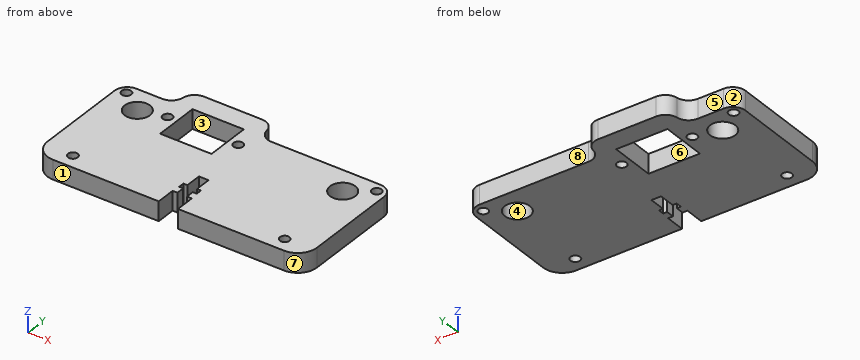
Autodesk Inventor part; units mm, degrees
ref_plane "YZ Plane" through (0, 0, 0) normal (1, 0, 0) x (0, 1, 0)
ref_plane "XZ Plane" through (0, 0, 0) normal (0, 1, 0) x (-1, 0, 0)
ref_plane "XY Plane" through (0, 0, 0) normal (0, 0, 1) x (1, 0, 0)
sketch "Sketch1" plane through (0, 0, 0) normal (0, 0, 1) x (1, 0, 0)
  arc A0 (-84, -33) -> (-78, -39) centre (-78, -33) ccw
  line L0 (-78, -39) -> (-45, -39)
  line L1 (-45, -39) -> (-45, -33)
  line L2 (-45, -33) -> (-43.5, -33)
  line L3 (-43.5, -33) -> (-43.5, -30.5)
  line L4 (-43.5, -30.5) -> (-44.75, -30.5)
  line L5 (-44.75, -30.5) -> (-44.75, -28.7)
  line L6 (-44.75, -28.7) -> (-43.5, -28.7)
  line L7 (-43.5, -28.7) -> (-43.5, -23.7)
  line L8 (-43.5, -23.7) -> (-40.5, -23.7)
  line L9 (-40.5, -23.7) -> (-40.5, -28.7)
  line L10 (-40.5, -28.7) -> (-39.25, -28.7)
  line L11 (-39.25, -28.7) -> (-39.25, -30.5)
  line L12 (-39.25, -30.5) -> (-40.5, -30.5)
  line L13 (-40.5, -30.5) -> (-40.5, -33)
  line L14 (-40.5, -33) -> (-39, -33)
  line L15 (-39, -33) -> (-39, -39)
  line L16 (-39, -39) -> (-6, -39)
  arc A1 (-6, -39) -> (0, -33) centre (-6, -33) ccw
  line L17 (0, -33) -> (0, -4)
  arc A2 (0, -4) -> (-4, 0) centre (-4, -4) ccw
  line L18 (-4, 0) -> (-38, 0)
  arc A3 (-41.9686, 3.5) -> (-38, 0) centre (-38, 4) ccw
  arc A4 (-41.9686, 3.5) -> (-45.9373, 7) centre (-45.9373, 3) ccw
  line L19 (-45.9373, 7) -> (-64.0627, 7)
  arc A5 (-64.0627, 7) -> (-68.0314, 3.5) centre (-64.0627, 3) ccw
  arc A6 (-72, 0) -> (-68.0314, 3.5) centre (-72, 4) ccw
  line L20 (-72, 0) -> (-80, 0)
  arc A7 (-80, 0) -> (-84, -4) centre (-80, -4) ccw
  line L21 (-84, -4) -> (-84, -33)
  line L22 (-63, 0.6) -> (-47, 0.6)
  line L23 (-47, 0.6) -> (-47, -13.4)
  line L24 (-47, -13.4) -> (-63, -13.4)
  line L25 (-63, -13.4) -> (-63, 0.6)
  circle A8 centre (-81, -3) radius 1.5
  circle A9 centre (-9, -34.5) radius 1.5
  circle A10 centre (-3, -3) radius 1.5
  circle A11 centre (-66, -6) radius 1.5
  circle A12 centre (-44, -6) radius 1.5
  circle A13 centre (-75, -34.5) radius 1.5
  circle A14 centre (-10, -8) radius 3.94
  circle A15 centre (-74, -8) radius 3.94
  point P0 (0, 0)
extrude "Extrusion1" add sketch "Sketch1" along normal blind 6
properties part number "XcrLeft_b"
Geometry: final body of the model. Coordinates: model frame, mm. Face numbers are marked on the shaded views. A direction names the side the tool comes from. Coordinates: 2 decimals unless noted, no trailing zeros. Order: outer loops, then holes, each group sorted by start corner. A loop starts at its lowest first (then second) coordinate and runs counter-clockwise, first axis right, second up. Notation, with made-up numbers: M 27.25,67 L 45.25,67 A24 ccw 45.25,104 Z; hole C -22,62.5 d5. An arc over 180 degrees is marked long. Answer in a Markdown table with one row per item. Add a question column.
Q1. Reachability of the marked faces 5, 6, 7 and 8 from +Z, -Z, +X, -X, +Y, -Y: full face, straight path, thin tool, end or side. Return the list, or none.
Q2. Contact query for flat-ended pins moving along their axis: P1, Ø1.2, axis at y = -31.5, z = 3, coming from the +X side; P2, Ø0.6, axis at x = -44, z = 3, coming from the -Y side; P3, Ø0.6, axis at x = -44, z = 3, coming from the +Y side. Output: stop coordinate, or through.
Q3. Section query D-D on z = 1.75. Count the separate pieces of the cut face and the enclosed holes in it, and give its area (3 significant figures).
Q4. Mould query, pull axis X, two halves, no side actions, for the marked faces 1, 2, 3 and 4. Classes: released by +X, released by -X, zero draft, split by the parting line, or undercut.
Q5. Line query: L1, parallel to X at y = -4, z = 3.75; L2, parallel to Y at x = -56, z = 0.7; L3, parallel to Y at x = -10, z = 2.45. Output: solid intervals per line, ascending.
Q6. Section query B-B on y = -3. Return the cut outline in (x, z), and give its area (3 significant figures).
Q7. Section query C-C on x = -75. Return the cut outline in (y, z).
Q8. Section query A-A on x = -59. Return the cut outline in (y, z), and give its area (3 significant figures).
Completed:
| question | item | result |
|---|---|---|
| 1 | face 5 | +Z, -Z, -X, +Y |
| 1 | face 6 | +Z, -Z |
| 1 | face 7 | +Z, -Z, +X, -Y |
| 1 | face 8 | +Z, -Z, +X, +Y |
| 2 | P1 | stops at x = 0 |
| 2 | P2 | stops at y = -33 |
| 2 | P3 | stops at y = 6.65 |
| 3 | separate pieces | 1 |
| 3 | enclosed holes | 9 |
| 3 | area | 3,000 mm2 |
| 4 | face 1 | zero draft |
| 4 | face 2 | released by -X |
| 4 | face 3 | undercut |
| 4 | face 4 | undercut |
| 5 | L1 | x = -84 to -82.12, -79.88 to -63, -47 to -4.12, -1.88 to 0 |
| 5 | L2 | y = -39 to -13.4, 0.6 to 7 |
| 5 | L3 | y = -39 to -35.62, -33.38 to -11.94, -4.06 to 0 |
| 6 | outline | M -83.87,0 L -82.5,0 L -82.5,6 L -83.87,6 Z; M -79.5,0 L -63,0 L -63,6 L -79.5,6 Z; M -47,0 L -4.5,0 L -4.5,6 L -47,6 Z; M -1.5,0 L -0.13,0 L -0.13,6 L -1.5,6 Z |
| 6 | area | 370 mm2 |
| 7 | outline | M -39,0 L -36,0 L -36,6 L -39,6 Z; M -33,0 L -11.81,0 L -11.81,6 L -33,6 Z; M -4.19,0 L 0,0 L 0,6 L -4.19,6 Z |
| 8 | outline | M -39,0 L -13.4,0 L -13.4,6 L -39,6 Z; M 0.6,0 L 7,0 L 7,6 L 0.6,6 Z |
| 8 | area | 192 mm2 |
